from build123d import *

# Parameters (mm, degrees)
F0_W     = 32
F0_H     = 10
F1_DEPTH = 1.5
F2_W     = 4
F2_H     = 10
F3_DEPTH = 8
F4_R     = 2.5
F5_DEPTH = 50
F6_R     = 2.5
F6_R_2   = 1.75
F7_DEPTH = 3
F8_R     = 2.5
F8_R_2   = 1.75
F9_DEPTH = 3


with BuildPart() as f1:
    # F0 (on Top) → F1 (new body)
    with BuildSketch(Plane.XY):
        Rectangle(F0_W, F0_H)
    extrude(amount=F1_DEPTH)

    # F2 (on face) → F3 (join)
    with BuildSketch(Plane.XY.offset(1.5)):
        with Locations((-16, 0)):
            Rectangle(F2_W, F2_H)
        with Locations((16, 0)):
            Rectangle(F2_W, F2_H)
    extrude(amount=F3_DEPTH)

    # F4 (on face) → F5 (cut)
    with BuildSketch(Plane(origin=(-18, 0, 0), x_dir=(0, -1, 0), z_dir=(-1, 0, 0))):
        with Locations((0, 5.397753)):
            Circle(F4_R)
    extrude(amount=-F5_DEPTH, mode=Mode.SUBTRACT)

    # F6 (on face) → F7 (join)
    with BuildSketch(Plane(origin=(-18, 0, 0), x_dir=(0, -1, 0), z_dir=(-1, 0, 0))):
        with Locations((0, 5.397753)):
            Circle(F6_R)
        with Locations((0, 5.397753)):
            Circle(F6_R_2, mode=Mode.SUBTRACT)
    extrude(amount=-F7_DEPTH)

    # F8 (on face) → F9 (join)
    with BuildSketch(Plane.YZ.offset(18)):
        with Locations((0, 5.397753)):
            Circle(F8_R)
        with Locations((0, 5.397753)):
            Circle(F8_R_2, mode=Mode.SUBTRACT)
    extrude(amount=-F9_DEPTH)


solid = f1.part
Part model, mm, in its own coordinate system. A direction names the side the tool comes from. Coordinates: 2 decimals unless noted, no trailing zeros. Order: outer loops, then holes, each group sorted by start corner. A loop starts at its lowest first (then second) coordinate and runs counter-clockwise, first axis right, second up. Notation, with made-up numbers: (83.25, 50.5) - (122.25, 50.5) arc R13 ccw to (122.25, 70.5) - close; hole circle Ø11 at (21.5, 4.5). An arc over 180 degrees is marked (long way). Use CSV: the item, a comma, the result in double quotes.
Item 1: Saw through at C-C on y = 4. Give the cut face in (x, z), and give its area (3 significant figures).
Solved:
outline,"(-18, 1.5) - (-16, 1.5) - (-16, 0) - (16, 0) - (16, 1.5) - (18, 1.5) - (18, 9.5) - (14, 9.5) - (14, 1.5) - (-14, 1.5) - (-14, 9.5) - (-18, 9.5) - close"
area,"112 mm²"
Item 2: Saw through at B-B on y = 0. Give the cut face in (x, z).
Solved:
outline,"(-18, 1.5) - (-16, 1.5) - (-16, 0) - (16, 0) - (16, 1.5) - (18, 1.5) - (18, 3.65) - (15, 3.65) - (15, 2.9) - (14, 2.9) - (14, 1.5) - (-14, 1.5) - (-14, 2.9) - (-15, 2.9) - (-15, 3.65) - (-18, 3.65) - close; (-18, 7.15) - (-15, 7.15) - (-15, 7.9) - (-14, 7.9) - (-14, 9.5) - (-18, 9.5) - close; (14, 7.9) - (15, 7.9) - (15, 7.15) - (18, 7.15) - (18, 9.5) - (14, 9.5) - close"
Item 3: Saw through at D-D on z = 4. Give the cut face in (x, y), and give its area (3 significant figures).
Solved:
outline,"(-18, -5) - (-14, -5) - (-14, -2.07) - (-15, -2.07) - (-15, -1.05) - (-18, -1.05) - close; (-18, 1.05) - (-15, 1.05) - (-15, 2.07) - (-14, 2.07) - (-14, 5) - (-18, 5) - close; (14, -5) - (18, -5) - (18, -1.05) - (15, -1.05) - (15, -2.07) - (14, -2.07) - close; (14, 2.07) - (15, 2.07) - (15, 1.05) - (18, 1.05) - (18, 5) - (14, 5) - close"
area,"59.1 mm²"
Item 4: 3-axis set-ups, long thin cutter, end or side, ignore diameter. For faces 5 (the face through (-16, 0, 1)), 6 (the face through (17, 0, 1.5)), 7 (the face through (-14, -0.1, 8.1)), 8 (the face through (-18, 0.1, 7.3)), 9 (the face through (14.493, 0.325, 7.876)): which of +Z, -Z, +X, -X, +Y, -Y reach the whole face in a straight line?
Solved:
face 5,"-Z, -X, +Y, -Y"
face 6,"-Z, +X, +Y, -Y"
face 7,"+Z, +Y, -Y"
face 8,"+Z, -Z, -X, +Y, -Y"
face 9,"none"
Item 5: Drop flat-ended pins along their axis: P1, Ø3, axis at y = 0, z = 5.4, coming from the +X side; P2, Ø2, axis at x = -17.5, y = 2, coming from the -Z side; P3, Ø2, axis at x = -7.5, y = -3.5, coming from the +Z side; P4, Ø1.2, axis at y = -1.5, z = 0.5, coming from the -X side. Give the stop position or say it passes through.
Solved:
P1,"passes through"
P2,"stops at z = 1.5"
P3,"stops at z = 1.5"
P4,"stops at x = -16"
Item 6: Mould opens along Z. For faces 1 (the face through (1, 5, 1)), 2 (the face through (0, 0, 0)), 3 (the face through (16.521, -0.228, 7.133)), 4 (the face through (0, 0, 1.5)) say: +Z half, -Z half, draft (parallel to the pull), parting line (faces both ways), or undercut.
Solved:
face 1,"draft"
face 2,"-Z half"
face 3,"undercut"
face 4,"+Z half"
Item 7: Saw through at A-A on z = 9. Give the cut face in (x, y), and give its area (3 significant figures).
Solved:
outline,"(-18, -5) - (-14, -5) - (-14, 5) - (-18, 5) - close; (14, -5) - (18, -5) - (18, 5) - (14, 5) - close"
area,"80.0 mm²"
Item 8: Probe probe 1 along X at (y, z) = (1.75, 3.5); probe 2 along Z at (x, y) = (16.45, 0); probe 3 along Z at (x, y) = (-14.6, 0). List the from-to ranges inside material, lowest first.
Solved:
probe 1,"x = -18 to -14, 14 to 18"
probe 2,"z = 1.5 to 3.65, 7.15 to 9.5"
probe 3,"z = 0 to 2.9, 7.9 to 9.5"
